from build123d import *

# Parameters (mm, degrees)
SCHIZZO2_R                      = 67
ESTRUSIONE_ESTRUSIONE1_DEPTH    = 7
SCHIZZO3_R                      = 2
TAGLIO_ESTRUSIONE2_DEPTH        = 7
RIPETIZIONECIRCOLARE1_COUNT     = 4
FORO_FILETTATO_M3_1_D           = 2.5
FORO_FILETTATO_M3_1_CSINK_D     = 3.05
FORO_FILETTATO_M3_1_CSINK_ANGLE = 90
SCHIZZO4_R                      = 50
TAGLIO_ESTRUSIONE3_DEPTH        = 7


with BuildPart() as part:
    # Schizzo2 → Estrusione-Estrusione1 (new body)
    with BuildSketch(Plane.XY):
        Circle(SCHIZZO2_R)
    extrude(amount=ESTRUSIONE_ESTRUSIONE1_DEPTH)

    # Schizzo3 → Taglio-Estrusione2 (cut)
    with BuildSketch(Plane.XY):
        with Locations(Location((0, 62, 0), (0, 0, 180))):
            Circle(SCHIZZO3_R)
    taglio_estrusione2 = extrude(amount=TAGLIO_ESTRUSIONE2_DEPTH, mode=Mode.SUBTRACT)

    # RipetizioneCircolare1: Taglio-Estrusione2 ×4 about axis
    ripetizionecircolare1_axis = Axis((0, 0, 0), (0, 0, 1))
    for i in range(1, RIPETIZIONECIRCOLARE1_COUNT):
        add(taglio_estrusione2.rotate(ripetizionecircolare1_axis, i * 360 / RIPETIZIONECIRCOLARE1_COUNT), mode=Mode.SUBTRACT)

    # Foro filettato M3-1 (through all)
    with Locations(Plane(origin=(-42.39, -36.56, 7), x_dir=(1, 0, 0), z_dir=(0, 0, 1))):
        with Locations((0, 0), (84.78, 0), (84.78, 73.12), (0, 73.12)):
            CounterSinkHole(FORO_FILETTATO_M3_1_D / 2, FORO_FILETTATO_M3_1_CSINK_D / 2, counter_sink_angle=FORO_FILETTATO_M3_1_CSINK_ANGLE)

    # Schizzo4 → Taglio-Estrusione3 (cut)
    with BuildSketch(Plane.XY.offset(7)):
        Circle(SCHIZZO4_R)
    extrude(amount=-TAGLIO_ESTRUSIONE3_DEPTH, mode=Mode.SUBTRACT)


solid = part.part
Source: CAD feature listing. Evaluate the final solid. Frame: model axes, mm. Coordinates: 2 decimals unless noted, no trailing zeros. Loops run counter-clockwise (first coordinate to the right, second up) from the corner with the lowest first, then second, coordinate; pieces in that order, holes last. Notation, with made-up numbers: M -34,-32 L -5,-32 A27 ccw -5,-5 Z; hole C 28,76 d2. An arc over 180 degrees is marked long. Answer in a Markdown table with one row per item.
Q1. Section A-A on z = 2. State how many separate pieces and enclosed holes the cut face has, plus the area to 3 significant figures.
Answers below:
| item | result |
|---|---|
| separate pieces | 1 |
| enclosed holes | 9 |
| area | 6,180 mm^2 |
Q2. Draft query along Y for faces 1 (the flat face through (-50, -5, 7)), 2 (the cylindrical face through (0, -60, 3)), 3 (the cylindrical face through (-14.524, -65.407, 3.451)), 4 (the cylindrical face through (47.69, 15.02, 3.55)). Return one class per face: pulls with the +Y half, pulls with the -Y half, needs draft (parallel to the pull), parting line crosses it, or undercut.
Answers below:
| item | result |
|---|---|
| face 1 | needs draft |
| face 2 | undercut |
| face 3 | parting line crosses it |
| face 4 | undercut |
Q3. First-contact query: pin 1 (4 mm diameter, centred on x = -2.5, z = 5, fed in from -Y); pin 2 (5 mm diameter, centred on x = 0, y = -62, fed in from -Z); pin 3 (2 mm diameter, centred on y = -8, z = 1, fed in from -X); pin 4 (2 mm diameter, centred on x = 19, z = 5.5, fed in from -Y). Flat tips, straight axial feed; report the tip coordinate or a pass-through.
Answers below:
| item | result |
|---|---|
| pin 1 | stops at y = -67 |
| pin 2 | stops at z = 0 |
| pin 3 | stops at x = -66.63 |
| pin 4 | stops at y = -64.54 |
Q4. Section B-B on y = 0. Return the cut outline in (x, z).
Answers below:
| item | result |
|---|---|
| outline | M -67,0 L -64,0 L -64,7 L -67,7 Z; M -60,0 L -50,0 L -50,7 L -60,7 Z; M 50,0 L 60,0 L 60,7 L 50,7 Z; M 64,0 L 67,0 L 67,7 L 64,7 Z |
Q5. Section D-D on y = -62. Return the cut outline in (x, z), plus the area to 3 significant figures.
Answers below:
| item | result |
|---|---|
| outline | M -25.4,0 L -2,0 L -2,7 L -25.4,7 Z; M 2,0 L 25.4,0 L 25.4,7 L 2,7 Z |
| area | 328 mm^2 |
Q6. Ray query, probe 1 along Y at (x, z) = (0, 3.25); probe 2 along X at (y, z) = (0.5, 4.25); probe 3 along X at (y, z) = (-37.5, 0.75). Return the intervals inside material, ascending. Write a range as from..to.
Answers below:
| item | result |
|---|---|
| probe 1 | y = -67..-64, -60..-50, 50..60, 64..67 |
| probe 2 | x = -67..-63.94, -60.06..-50, 50..60.06, 63.94..67 |
| probe 3 | x = -55.52..-43.21, -41.57..-33.07, 33.07..41.57, 43.21..55.52 |
